from build123d import *

# Parameters (mm, degrees)
RESSALTO_EXTRUS_O1_DEPTH   = 5
CORTE_EXTRUS_O1_START      = -10
CORTE_EXTRUS_O1_DEPTH      = 7.866546
ESBO_O4_R                  = 1.75
CORTE_EXTRUS_O2_DEPTH      = 21.366546328
ESBO_O5_R                  = 1.75
CORTE_EXTRUS_O3_DEPTH      = 2.5
CORTE_EXTRUS_O3_DEPTH_BACK = 13.5
ESBO_O6_W                  = 10
ESBO_O6_H                  = 7.25
RESSALTO_EXTRUS_O2_DEPTH   = 0.5
ESBO_O6_2_R                = 1.75
CORTE_EXTRUS_O4_DEPTH      = 1.5
CORTE_EXTRUS_O4_DEPTH_BACK = 1


with BuildPart() as part:
    # Esboço1 → Ressalto-extrusão1 (new body, symmetric)
    with BuildSketch(Plane.XY):
        with BuildLine():
            Line((-4, 0), (4, 0))
            Line((4, 0), (4, 4.505437353))
            ThreePointArc((4, 4.505437353), (6.923679872, 9.219147423), (5.5, 14.580127019))
            Line((5.5, 14.580127019), (5.5, 20.366546328))
            Line((5.5, 20.366546328), (2.5, 20.366546328))
            Line((2.5, 20.366546328), (2.5, 14.866546328))
            ThreePointArc((2.5, 14.866546328), (0, 5), (-2.5, 14.866546328))
            Line((-2.5, 14.866546328), (-2.5, 20.366546328))
            Line((-2.5, 20.366546328), (-5.5, 20.366546328))
            Line((-5.5, 20.366546328), (-5.5, 14.580127019))
            ThreePointArc((-5.5, 14.580127019), (-6.923679872, 9.219147423), (-4, 4.505437353))
            Line((-4, 4.505437353), (-4, 0))
        make_face()
    extrude(amount=RESSALTO_EXTRUS_O1_DEPTH, both=True)

    # Esboço3 → Corte-extrusão1 (cut)
    with BuildSketch(Plane(origin=(0, 20.366546328, 0), x_dir=(1, 0, 0), z_dir=(0, 1, 0)).offset(CORTE_EXTRUS_O1_START)):
        Polygon((0, 3.233161507), (-2.8, 1.616580754), (-2.8, -1.616580754), (0, -3.233161507), (2.8, -1.616580754), (2.8, 1.616580754), align=None)
    extrude(amount=-CORTE_EXTRUS_O1_DEPTH, mode=Mode.SUBTRACT)

    # Esboço4 → Corte-extrusão2 (cut, through all)
    with BuildSketch(Plane(origin=(0, 20.366546328, 0), x_dir=(1, 0, 0), z_dir=(0, 1, 0))):
        Circle(ESBO_O4_R)
    extrude(amount=-CORTE_EXTRUS_O2_DEPTH, mode=Mode.SUBTRACT)

    # Esboço5 → Corte-extrusão3 (cut, two sides)
    with BuildSketch(Plane(origin=(5.5, 0, 0), x_dir=(0, 0, -1), z_dir=(1, 0, 0))) as corte_extrus_o3_sk:
        with Locations((0, 17.116546328)):
            Circle(ESBO_O5_R)
    extrude(amount=CORTE_EXTRUS_O3_DEPTH, mode=Mode.SUBTRACT)
    extrude(corte_extrus_o3_sk.sketch, amount=-CORTE_EXTRUS_O3_DEPTH_BACK, mode=Mode.SUBTRACT)

    # Esboço6 → Ressalto-extrusão2 (add)
    with BuildSketch(Plane.ZY.offset(5.5)):
        with Locations((0, 16.741546328)):
            Rectangle(ESBO_O6_W, ESBO_O6_H)
        Polygon((3.233161507, 17.116546328), (1.616580754, 19.916546328), (-1.616580754, 19.916546328), (-3.233161507, 17.116546328), (-1.616580754, 14.316546328), (1.616580754, 14.316546328), align=None, mode=Mode.SUBTRACT)
    extrude(amount=RESSALTO_EXTRUS_O2_DEPTH)

    # Esboço6<2> → Corte-extrusão4 (cut, two sides)
    with BuildSketch(Plane.ZY.offset(5.5)) as corte_extrus_o4_sk:
        Polygon((-3.233161507, 17.116546328), (-1.768759136, 14.580127019), (1.768759136, 14.580127019), (3.233161507, 17.116546328), (1.616580754, 19.916546328), (-1.616580754, 19.916546328), align=None)
        with Locations((0, 17.116546328)):
            Circle(ESBO_O6_2_R, mode=Mode.SUBTRACT)
        Polygon((1.768759136, 14.580127019), (-1.768759136, 14.580127019), (-1.616580754, 14.316546328), (1.616580754, 14.316546328), align=None)
    extrude(amount=CORTE_EXTRUS_O4_DEPTH, mode=Mode.SUBTRACT)
    extrude(corte_extrus_o4_sk.sketch, amount=-CORTE_EXTRUS_O4_DEPTH_BACK, mode=Mode.SUBTRACT)


solid = part.part
Design review of the part built by this model. Coordinates are the model's own, in mm. A direction names the side the tool comes from. Give positions to 0.01 mm unless a question says otherwise; leave off trailing zeros. Loops run counter-clockwise (first coordinate to the right, second up) from the corner with the lowest first, then second, coordinate; pieces in that order, holes last. Notation, with made-up numbers: (81.5, 89) -> (113.5, 89) arc R29 cw to (113.5, 122) -> close; hole circle Ø9 at (-22.75, 12.5). An arc over 180 degrees is marked (long way). One line per question, with ' | ' between items. Start each with the question number.
(1) Draft analysis for pull direction Y (two halves, no side actions). For faces 5 (the face through (-5, 19.917, 0)), 6 (the face through (5.5, 19, 1)), 7 (the face through (-2, 0, 0)), state which applies: +Y half, -Y half, draft (parallel to the pull), parting line (faces both ways), or undercut.
(2) Insertion check: P1, Ø4.5, axis at y = 17.12, z = 0, coming from the +X side; P2, Ø4.5, axis at y = 18.5, z = -0.5, coming from the -X side; P3, Ø1.4, axis at y = 1, z = -1.5, coming from the -X side. Each pin has a flat end and moves straight along its axis. Give the tip position at first contact, or say it passes through.
(3) We need section C-C (x = 4.75). State the section outline as (y, z) points.
(4) For line 1 (X direction, y = 16.25, z = -2.5); line 2 (Y direction, x = 2.75, z = -1.25); line 3 (X direction, y = 16, z = 4), list the stretches that pass through material, from the lowest coordinate up.
(5) We need section A-A (z = 0). State how many separate pieces and enclosed holes the cut face has, and give its area (3 significant figures).
(6) We need section B-B (y = 10.25). State the section outline as (x, z) points, and give its area (3 significant figures).
(7) We need section D-D (z = 4). State the section outline as (x, y) points, and give its area (3 significant figures).
(8) For faces 1 (the face through (4, 2, 0)), 2 (the face through (-1.3, 2.5, 1.4)), 3 (the face through (-4.5, 19.02, -0.05)), 4 (the face through (2.5, 19, 1)), list the 3-axis set-ups (+Z, -Z, +X, -X, +Y, -Y) from which the entire face can be reached by the end or side of a thin tool; tool diameter is ignored.
The answers:
1) face 5: undercut | face 6: draft | face 7: -Y half
2) P1: stops at x = 5.5 | P2: stops at x = -6 | P3: stops at x = -4
3) outline: (5.11, -5) -> (8.01, -5) -> (8.01, 5) -> (5.11, 5) -> close; (12.49, -5) -> (20.37, -5) -> (20.37, 5) -> (12.49, 5) -> close; hole circle Ø3.5 at (17.12, 0)
4) line 1: x = -4.5 to -2.5, 2.5 to 5.5 | line 2: y = 0 to 2.5, 14.72 to 15.89, 18.34 to 20.37 | line 3: x = -6 to -2.5, 2.5 to 5.5
5) separate pieces: 4 | enclosed holes: 0 | area: 67.3 mm^2
6) outline: (-7, -5) -> (-5.25, -5) -> (-5.25, 5) -> (-7, 5) -> close; (5.25, -5) -> (7, -5) -> (7, 5) -> (5.25, 5) -> close | area: 35.0 mm^2
7) outline: (-6, 13.86) arc R7 ccw to (-4, 4.51) -> (-4, 0) -> (4, 0) -> (4, 4.51) arc R7 ccw to (5.5, 14.58) -> (5.5, 20.37) -> (2.5, 20.37) -> (2.5, 14.87) arc R5.25 cw (long way) to (-2.5, 14.87) -> (-2.5, 20.37) -> (-6, 20.37) -> close | area: 117 mm^2
8) face 1: +Z, -Z, +X, -Y | face 2: none | face 3: -X | face 4: +Z, -Z, +Y
